```python
from build123d import *

# Parameters (mm, degrees)
BOSS_EXTRUDE1_DEPTH      = 3.175
BOSS_EXTRUDE1_DEPTH_BACK = 3.175
CHAMFER1_SIZE            = 20
FILLET1_R                = 15
FILLET2_R                = 3
SKETCH4_W                = 3.175
SKETCH4_H                = 50
SKETCH4_W_2              = 15
SKETCH4_H_2              = 3.175
SKETCH4_W_3              = 100
SKETCH4_H_3              = 100
WALL_SLOTS_DEPTH         = 60
FILLET3_R                = 3


with BuildPart() as part:
    # Sketch2 → Boss-Extrude1 (new body, two sides)
    with BuildSketch(Plane.XY) as boss_extrude1_sk:
        Polygon((-157.4125, 94.825), (-107.4125, 94.825), (-107.4125, 0), (107.4125, 0), (107.4125, 209.825), (183.7625, 209.825), (183.7625, -76.35), (58.275, -76.35), (-31.925, -76.35), (-157.4125, -76.35), align=None)
    extrude(amount=BOSS_EXTRUDE1_DEPTH)
    extrude(boss_extrude1_sk.sketch, amount=-BOSS_EXTRUDE1_DEPTH_BACK)

    # Chamfer1
    chamfer1_edges = [part.edges().sort_by_distance(p)[0] for p in [
        (-157.4125, 94.825, 0),
        (183.7625, 209.825, 0),
        (183.7625, -76.35, 0),
        (-157.4125, -76.35, 0),
    ]]
    chamfer(chamfer1_edges, length=CHAMFER1_SIZE)

    # Fillet1
    fillet1_edges = [part.edges().sort_by_distance(p)[0] for p in [
        (-107.4125, 0, 0),
        (107.4125, 0, 0),
    ]]
    fillet(fillet1_edges, radius=FILLET1_R)

    # Fillet2
    fillet2_edges = [part.edges().sort_by_distance(p)[0] for p in [
        (-107.4125, 94.825, 0),
        (107.4125, 209.825, 0),
        (-157.4125, 74.825, 0),
        (-157.4125, -56.35, 0),
        (183.7625, 189.825, 0),
        (183.7625, -56.35, 0),
        (163.7625, 209.825, 0),
        (-137.4125, 94.825, 0),
    ]]
    fillet(fillet2_edges, radius=FILLET2_R)

    # Sketch4 → wall_slots (cut)
    with BuildSketch(Plane.XY.offset(3.175)):
        with Locations((-109, 53.4125)):
            Rectangle(SKETCH4_W, SKETCH4_H)
        with Locations((-123.291179656, 93.2375)):
            Rectangle(SKETCH4_W_2, SKETCH4_H_2)
        Polygon((-142.109199141, 90.128300859), (-152.715800859, 79.521699141), (-150.470736829, 77.276635111), (-139.864135111, 87.883236829), align=None)
        with Locations((-155.825, 9.2375)):
            Rectangle(SKETCH4_W, SKETCH4_H)
        Polygon((-150.031397, -59.240974939), (-152.276461031, -61.486038969), (-141.669859313, -72.092640687), (-139.424795283, -69.847576657), align=None)
        with Locations((13.175, -74.7625)):
            Rectangle(SKETCH4_W_3, SKETCH4_H_2)
        with Locations((0, -1.5875)):
            Rectangle(SKETCH4_W_3, SKETCH4_H_2)
        Polygon((165.774795283, -69.847576657), (168.019859313, -72.092640687), (173.323160172, -66.789339828), (171.078096142, -64.544275798), align=None)
        Polygon((171.078096142, -64.544275798), (173.323160172, -66.789339828), (178.626461031, -61.486038969), (176.381397, -59.240974939), align=None)
        with Locations((182.175, 66.7375)):
            Rectangle(SKETCH4_W, SKETCH4_H_3)
        with Locations((109, 110.9125)):
            Rectangle(SKETCH4_W, SKETCH4_H_3)
        with Locations((136.466179656, 208.2375)):
            Rectangle(SKETCH4_W_2, SKETCH4_H_2)
        Polygon((179.065800859, 194.521699141), (168.459199141, 205.128300859), (166.214135111, 202.883236829), (176.820736829, 192.276635111), align=None)
    extrude(amount=-WALL_SLOTS_DEPTH, mode=Mode.SUBTRACT)

    # Fillet3
    fillet3_edges = [part.edges().sort_by_distance(p)[0] for p in [
        (163.7625, -76.35, 0),
        (-137.4125, -76.35, 0),
    ]]
    fillet(fillet3_edges, radius=FILLET3_R)


solid = part.part
```
Design review of the part built by this model. Coordinates are the model's own, in mm. A direction names the side the tool comes from. Give positions to 0.01 mm unless a question says otherwise; leave off trailing zeros. Order: outer loops, then holes, each group sorted by start corner. A loop starts at its lowest first (then second) coordinate and runs counter-clockwise, first axis right, second up. Notation, with made-up numbers: (2, 77.25) - (11, 77.25) arc R31 ccw to (11, 101.25) - close; hole circle Ø4 at (66, 68). An arc over 180 degrees is marked (long way). Use a Markdown table: item, result. Add a question column.
(1) Add section A-A on y = 166.5. Give the boundary of the cut face in (x, z) (1 decimal), then the cut area to 3 significant figures.
(2) Machinability: for faces 1 (the face through (-144.65, -64.62, 0.04)), 2 (the face through (102.902, 4.277, -0.044)), 3 (the face through (53, -27, 3.175)), which of the approach directions +Z, -Z, +X, -X, +Y, -Y give a long, thin tool a straight path to every point of the face, cutting with its end or side? Answer none if there is none.
(3) Clearance check with flat-ended pins moving along their axes: P1, Ø3, axis at y = 85.5, z = 0, coming from the +X side; P2, Ø2, axis at y = 84, z = -1, coming from the -X side; P3, Ø2.5, axis at x = -156, z = 1.5, coming from the -Y side. State where each tip first meets the part, or that it passes through.
(4) Wall thickness on probe 1 along X at (y, z) = (40, 0.5); probe 2 along X at (y, z) = (22.5, -1.25); probe 3 along X at (y, z) = (150.5, -1.25): over which ranges is each line inside the solid? List them lowest first. Write a range as [from, to].
(5) Add section B-B on x = -28. Give the boundary of the cut face in (y, z) (3 decimals).
(6) Mouldability with a two-part tool opening along Y and no side actions: class faces 4 (the face through (-103.135, 4.511, -0.044)), 5 (the face through (53, -27, -3.175)), 6 (the face through (-145.24, 82.51, 0.04)), 7 (the face through (171.4, 197.7, 0)) as +Y half, -Y half, draft (parallel to the pull), parting line (faces both ways), or undercut.
Report:
| question | item | result |
|---|---|---|
| 1 | outline | (107.4, -3.2) - (183.8, -3.2) - (183.8, 3.2) - (107.4, 3.2) - close |
| 1 | area | 485 mm² |
| 2 | face 1 | +Z, -Z |
| 2 | face 2 | +Z, -Z, +Y |
| 2 | face 3 | +Z, +X, -X, +Y, -Y |
| 3 | P1 | stops at x = 180.59 |
| 3 | P2 | stops at x = -144.75 |
| 3 | P3 | stops at y = -59.01 |
| 4 | probe 1 | x = [-157.41, -110.59], [107.41, 180.59] |
| 4 | probe 2 | x = [-154.24, -107.41], [107.41, 180.59] |
| 4 | probe 3 | x = [110.59, 183.76] |
| 5 | outline | (-73.175, -3.175) - (-3.175, -3.175) - (-3.175, 3.175) - (-73.175, 3.175) - close |
| 6 | face 4 | +Y half |
| 6 | face 5 | draft |
| 6 | face 6 | undercut |
| 6 | face 7 | undercut |
